For this review, take the finished solid that the model builds, in its own axes (mm). A direction names the side the tool comes from. Coordinates: 2 decimals unless noted, no trailing zeros. Write each loop counter-clockwise with the first axis right and the second up, starting at its lowest first coordinate (ties: lowest second). Pieces come first, ordered by that corner, then holes.
```python
from build123d import *

# Parameters (mm, degrees)
SKETCH1_W            = 100
SKETCH1_H            = 130
BOSS_EXTRUDE1_DEPTH  = 8
M5_CLEARANCE_HOLE1_D = 5.8
SKETCH6_R            = 20
CUT_EXTRUDE1_DEPTH   = 10
SKETCH9_W            = 40
SKETCH9_H            = 130
SKETCH9_W_2          = 10
BOSS_EXTRUDE2_DEPTH  = 8
M5_CLEARANCE_HOLE2_D = 5.8
SKETCH13_W           = 7
SKETCH13_H           = 130
BOSS_EXTRUDE3_DEPTH  = 10
SKETCH14_W           = 30
SKETCH14_H           = 20
BOSS_EXTRUDE4_DEPTH  = 10
FILLET1_R            = 10
FILLET2_R            = 5
CUT_EXTRUDE2_REACH   = 138.839


with BuildPart() as part:
    # Sketch1 → Boss-Extrude1 (new body)
    with BuildSketch(Plane.XY):
        Rectangle(SKETCH1_W, SKETCH1_H)
    extrude(amount=BOSS_EXTRUDE1_DEPTH)

    # M5 Clearance Hole1 (through all)
    with Locations(Plane.XY.offset(8)):
        with Locations((-40, 6), (40, 6), (-40, -56), (40, -56), (-23.55, 58), (23.55, 58), (-23.55, 10.9), (23.55, 10.9), (-10, -56), (10, -56)):
            Hole(M5_CLEARANCE_HOLE1_D / 2)

    # Sketch6 → Cut-Extrude1 (cut)
    with BuildSketch(Plane.XY.offset(8)):
        with Locations((0, 34.5)):
            Circle(SKETCH6_R)
    extrude(amount=-CUT_EXTRUDE1_DEPTH, mode=Mode.SUBTRACT)

    # Sketch9 → Boss-Extrude2 (add)
    with BuildSketch(Plane.XY.offset(8)):
        with Locations((-70, 0)):
            Rectangle(SKETCH9_W, SKETCH9_H)
        with Locations((55, 0)):
            Rectangle(SKETCH9_W_2, SKETCH9_H)
    extrude(amount=-BOSS_EXTRUDE2_DEPTH)

    # M5 Clearance Hole2 (through all)
    with Locations(Plane.XY.offset(8)):
        with Locations((-75, 6), (-75, -56)):
            Hole(M5_CLEARANCE_HOLE2_D / 2)

    # Sketch13 → Boss-Extrude3 (add)
    with BuildSketch(Plane(origin=(0, 0, 0), x_dir=(-1, 0, 0), z_dir=(0, 0, -1))):
        with Locations((-56.5, 0)):
            Rectangle(SKETCH13_W, SKETCH13_H)
        with Locations((86.5, 0)):
            Rectangle(SKETCH13_W, SKETCH13_H)
    extrude(amount=BOSS_EXTRUDE3_DEPTH)

    # Sketch14 → Boss-Extrude4 (add)
    with BuildSketch(Plane.XY.offset(8)):
        with Locations((-105, 6)):
            Rectangle(SKETCH14_W, SKETCH14_H)
    extrude(amount=-BOSS_EXTRUDE4_DEPTH)

    # Fillet1
    fillet1_edges = [part.edges().sort_by_distance(p)[0] for p in [
        (-90, 16, 3),
        (-90, -4, 3),
    ]]
    fillet(fillet1_edges, radius=FILLET1_R)

    # Fillet2
    fillet2_edges = [part.edges().sort_by_distance(p)[0] for p in [
        (-120, -4, 3),
        (-120, 16, 3),
    ]]
    fillet(fillet2_edges, radius=FILLET2_R)

    # Sketch15 → Cut-Extrude2 (cut, up to next)
    with BuildSketch(Plane(origin=(0, 0, -2), x_dir=(-1, 0, 0), z_dir=(0, 0, -1)), mode=Mode.PRIVATE) as cut_extrude2_sk1:
        with BuildLine():
            Line((106, 16), (110, 16))
            ThreePointArc((110, 16), (108, 14), (106, 16))
        make_face()
    cut_extrude2_tool1 = extrude(cut_extrude2_sk1.sketch, amount=-CUT_EXTRUDE2_REACH, mode=Mode.PRIVATE) & part.part
    # Sketch15 → Cut-Extrude2 (cut, up to next)
    with BuildSketch(Plane(origin=(0, 0, -2), x_dir=(-1, 0, 0), z_dir=(0, 0, -1)), mode=Mode.PRIVATE) as cut_extrude2_sk2:
        with BuildLine():
            Line((110, -4), (106, -4))
            ThreePointArc((106, -4), (108, -2), (110, -4))
        make_face()
    cut_extrude2_tool2 = extrude(cut_extrude2_sk2.sketch, amount=-CUT_EXTRUDE2_REACH, mode=Mode.PRIVATE) & part.part
    add(cut_extrude2_tool1.solids().sort_by_distance((-108, 15.151174, -2))[0], mode=Mode.SUBTRACT)
    add(cut_extrude2_tool2.solids().sort_by_distance((-108, -3.151174, -2))[0], mode=Mode.SUBTRACT)


solid = part.part
```
Q1. Clearance check with flat-ended pins moving along their axes: pin 1 Ø6.5 at (x, y) = (40, 6) entering from -Z; pin 2 Ø5.5 at (x, z) = (-112, 3.5) entering from -Y; pin 3 Ø7.5 at (x, y) = (-75, -56) entering from +Z; pin 4 Ø24 at (x, y) = (-110.5, 3.5) entering from -Z. State where each tip first meets the part, or that it passes through.
Ans:
pin 1: stops at z = 0
pin 2: stops at y = -4
pin 3: stops at z = 8
pin 4: stops at z = -2
Q2. Draft analysis for pull direction Y (two halves, no side actions). For faces 6 (the cylindrical face through (-9.37, -58.83, 3.94)), 7 (the cylindrical face through (-119, -2, 3)), 8 (the flat face through (-14, 65, 5)), 9 (the flat face through (-86, 1, -10)), state which applies: +Y half, -Y half, draft (parallel to the pull), parting line (faces both ways), or undercut.
Ans:
face 6: undercut
face 7: -Y half
face 8: +Y half
face 9: draft
Q3. Add section D-D (x = 0). State the section outline as (y, z) points.
Ans:
outline: (-65, 0) - (14.5, 0) - (14.5, 8) - (-65, 8) - close; (54.5, 0) - (65, 0) - (65, 8) - (54.5, 8) - close
Q4. Add section A-A (x = 23.55). State the section outline as (y, z) points.
Ans:
outline: (-65, 0) - (8, 0) - (8, 8) - (-65, 8) - close; (13.8, 0) - (55.1, 0) - (55.1, 8) - (13.8, 8) - close; (60.9, 0) - (65, 0) - (65, 8) - (60.9, 8) - close
Q5. Tool access review of faces 1 (the flat face through (-113, -4, 3)), 2 (the flat face through (-11, 1, 8)), 3 (the flat face through (53, -1, -5)), 4 (the flat face through (-103, 16, 3)), 5 (the flat face through (-105, 6, -2)): name each direction out of +Z, -Z, +X, -X, +Y, -Y from which nothing blocks a thin tool from reaching the whole face with its end or side.
Ans:
face 1: +Z, -Z, -X, -Y
face 2: +Z, +X, -X, +Y, -Y
face 3: -Z, +Y, -Y
face 4: +Z, -Z, -X, +Y
face 5: -Z, -X, +Y, -Y
Q6. Add section B-B (y = 58). State the section outline as (x, z) points, then the cut area to 3 significant figures.
Ans:
outline: (-90, -10) - (-83, -10) - (-83, 0) - (-26.45, 0) - (-26.45, 8) - (-90, 8) - close; (-20.65, 0) - (20.65, 0) - (20.65, 8) - (-20.65, 8) - close; (26.45, 0) - (53, 0) - (53, -10) - (60, -10) - (60, 8) - (26.45, 8) - close
area: 1,250 mm2
Q7. For probe 1 along Y at (x, z) = (-75, 4.25); probe 2 along X at (y, z) = (-41, -0.75); probe 3 along Y at (x, z) = (-23.55, 4.25), list the stretches that pass through material, from the lowest coordinate up.
Ans:
probe 1: y = -65 to -58.9, -53.1 to 3.1, 8.9 to 65
probe 2: x = -90 to -83, 53 to 60
probe 3: y = -65 to 8, 13.8 to 55.1, 60.9 to 65
Q8. Add section C-C (z = -7.75). State the section outline as (x, y) points, then the cut area to 3 significant figures.
Ans:
outline: (-90, -65) - (-83, -65) - (-83, 65) - (-90, 65) - close; (53, -65) - (60, -65) - (60, 65) - (53, 65) - close
area: 1,820 mm2
